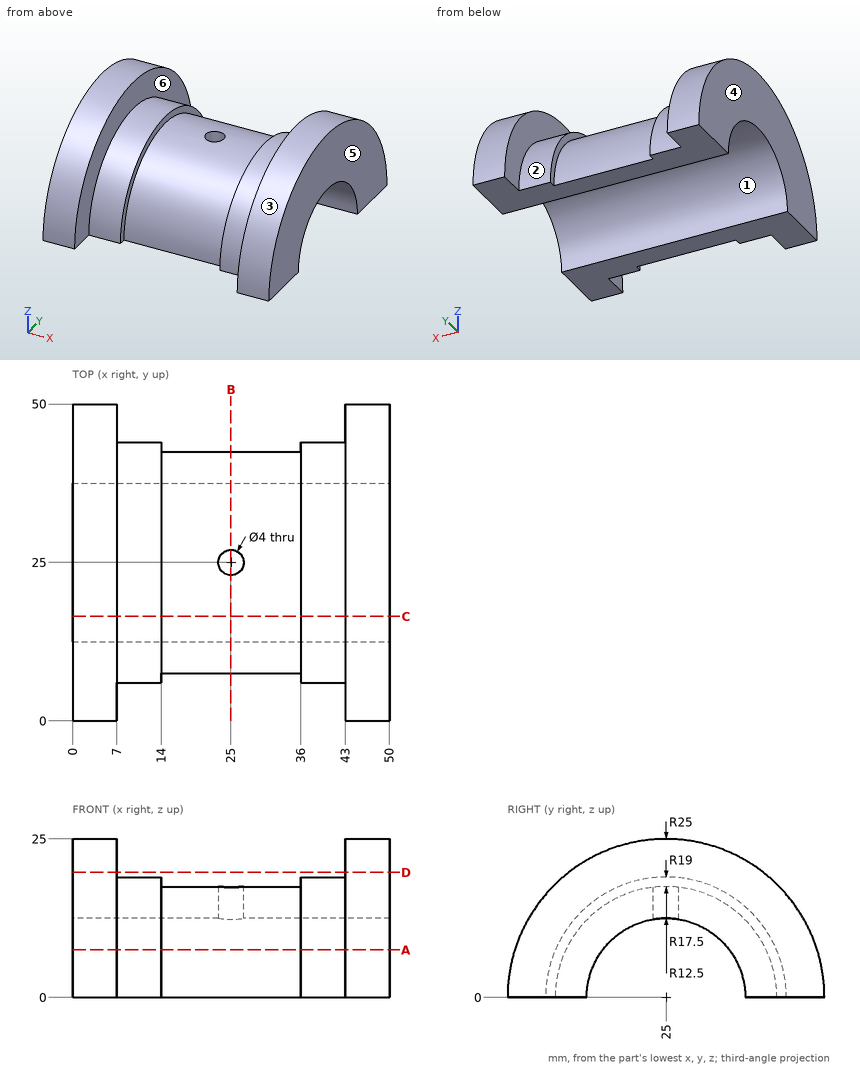
Job drawing, mm, ordinate dimensions from the low corner. One solid piece. A direction names the side the tool comes from. Coordinates: 2 decimals unless noted, no trailing zeros. Loops run counter-clockwise (first coordinate to the right, second up) from the corner with the lowest first, then second, coordinate; pieces in that order, holes last. Notation, with made-up numbers: (9.25, 22.5) - (23.25, 22.5) arc R7 cw to (23.25, 33.5) - close; hole circle Ø8 at (11.5, -18). An arc over 180 degrees is marked (long way). Answer as a JSON object with one key per item and string values. Group by question number.
(1) Cut at C-C (y = 16.5). Give the cut face in (x, z).
(2) Two-plate mould, pull along X, no slides. Class the marked faces 3, 4, 5 and 6: released by +X, released by -X, zero draft, split by the parting line, or undercut.
(3) Flat gauge pins, fed straight in: pin 1 (3 mm diameter, centred on x = 23.5, z = 19.5, fed in from +Y); pin 2 (2 mm diameter, centred on x = 25.5, z = 10, fed in from -Y); pin 3 (4 mm diameter, centred on x = 5.5, z = 13, fed in from +Y); pin 4 (12 mm diameter, centred on x = 5.5, z = 13.5, fed in from +Y). Where does each tip first touch, or does it go through?
(4) Probe line 1 along X through (y, z) = (25, 13.75); line 2 along X through (y, z) = (11, 11.5); line 3 along Y through (x, z) = (25, 13.6). List the from-to ranges inside material, lowest first.
(5) Cut at A-A (z = 7.5). Give the cut face in (x, y), then the cut area to 3 significant figures.
(6) Cut at D-D (z = 19.75). Give the cut face in (x, y).
(7) Cut at B-B (x = 25). Give the cut face in (y, z).
(8) Tool access for the marked faces 1 and 2: list every direction of +Z, -Z, +X, -X, +Y, -Y with a clear straight run to the whole face (end or side of a thin tool).
Geometry says:
{
 "1": {"outline": "(0, 9.17) - (50, 9.17) - (50, 23.51) - (43, 23.51) - (43, 16.99) - (36, 16.99) - (36, 15.3) - (14, 15.3) - (14, 16.99) - (7, 16.99) - (7, 23.51) - (0, 23.51) - close"},
 "2": {"face 3": "zero draft", "face 4": "released by -X", "face 5": "released by +X", "face 6": "undercut"},
 "3": {"pin 1": "passes through", "pin 2": "stops at y = 9.99", "pin 3": "stops at y = 47.45", "pin 4": "stops at y = 48.85"},
 "4": {"line 1": "x = 0 to 23, 27 to 50", "line 2": "x = 0 to 14, 36 to 50", "line 3": "y = 13.99 to 23, 27 to 36.01"},
 "5": {"outline": "(0, 1.15) - (7, 1.15) - (7, 7.54) - (14, 7.54) - (14, 9.19) - (36, 9.19) - (36, 7.54) - (43, 7.54) - (43, 1.15) - (50, 1.15) - (50, 15) - (0, 15) - close; (0, 35) - (50, 35) - (50, 48.85) - (43, 48.85) - (43, 42.46) - (36, 42.46) - (36, 40.81) - (14, 40.81) - (14, 42.46) - (7, 42.46) - (7, 48.85) - (0, 48.85) - close", "area": "852 mm^2"},
 "6": {"outline": "(0, 9.67) - (7, 9.67) - (7, 40.33) - (0, 40.33) - close; (43, 9.67) - (50, 9.67) - (50, 40.33) - (43, 40.33) - close"},
 "7": {"outline": "(7.5, 0) - (12.5, 0) arc R12.5 cw to (23, 12.34) - (23, 17.39) arc R17.5 ccw to start; (27, 12.34) arc R12.5 cw to (37.5, 0) - (42.5, 0) arc R17.5 ccw to (27, 17.39) - close"},
 "8": {"face 1": "-Z, +X, -X", "face 2": "+Z"}
}
